from build123d import *

# Parameters (mm, degrees)
F0_R     = 1.5
F1_DEPTH = 5
F2_W     = 5
F2_H     = 5
F2_H_2   = 4.5
F2_R     = 3.5
F3_DEPTH = 3
F4_R     = 1.5
F4_R_2   = 1.4524317573
F5_DEPTH = 25
F6_R     = 3
F7_DEPTH = 7
F8_SIZE  = 1.99999
F9_DEPTH = 25


# Not quite as in the source:
# - a fillet or chamfer is up to 0.001 mm smaller than in the source, because OpenCascade refuses the exact size


with BuildPart() as f1:
    # F0 (on Top) → F1 (new body)
    with BuildSketch(Plane.XY):
        with BuildLine():
            Line((100.4699678509, 5.9815658668), (2.0132142916, 17.3838133968))
            ThreePointArc((2.0132142916, 17.3838133968), (-17.4999985209, -0.0071949455), (2.027507963, -17.3821520952))
            Line((2.027507963, -17.3821520952), (99.6811939192, -5.991524237))
            ThreePointArc((99.6811939192, -5.991524237), (105.987022142, -0.394418396), (100.4699678509, 5.9815658668))
        make_face()
        with BuildLine():
            Line((-11, -8.6602540378), (-2.9686269666, -4.023338655))
            ThreePointArc((-2.9686269666, -4.023338655), (0, -5), (2.9686269666, -4.023338655))
            Line((2.9686269666, -4.023338655), (11, -8.6602540378))
            ThreePointArc((11, -8.6602540378), (0, -14), (-11, -8.6602540378))
        make_face(mode=Mode.SUBTRACT)
        with BuildLine():
            ThreePointArc((-13, -5.1961524227), (-12.124355653, 7), (-2, 13.8564064606))
            Line((-2, 13.8564064606), (-2, 4.582575695))
            ThreePointArc((-2, 4.582575695), (-4.3301270189, 2.5), (-4.9686269666, -0.5592370399))
            Line((-4.9686269666, -0.5592370399), (-13, -5.1961524227))
        make_face(mode=Mode.SUBTRACT)
        Circle(F0_R, mode=Mode.SUBTRACT)
        with BuildLine():
            Line((2, 4.582575695), (2, 13.8564064606))
            ThreePointArc((2, 13.8564064606), (12.124355653, 7), (13, -5.1961524227))
            Line((13, -5.1961524227), (4.9686269666, -0.5592370399))
            ThreePointArc((4.9686269666, -0.5592370399), (4.3301270189, 2.5), (2, 4.582575695))
        make_face(mode=Mode.SUBTRACT)
        with BuildLine():
            Line((30.3816278502, -10.0477205958), (13.8356347618, -11.9776963869))
            ThreePointArc((13.8356347618, -11.9776963869), (18.2999984533, 0.0075238573), (13.8257810711, 11.9890690954))
            Line((13.8257810711, 11.9890690954), (30.3733555452, 10.0726993863))
            ThreePointArc((30.3733555452, 10.0726993863), (31.9999972954, 0.0131564719), (30.3816278502, -10.0477205958))
        make_face(mode=Mode.SUBTRACT)
        with BuildLine():
            Line((67.7617245486, -5.6875905441), (44.2022623135, -8.435639061))
            ThreePointArc((44.2022623135, -8.435639061), (44.9999961967, 0.0185012885), (44.1953109176, 8.4719828198))
            Line((44.1953109176, 8.4719828198), (67.7570248516, 5.743307693))
            ThreePointArc((67.7570248516, 5.743307693), (67.9999942528, 0.0279575027), (67.7617245486, -5.6875905441))
        make_face(mode=Mode.SUBTRACT)
        Polygon((77.8001793809, -5), (77.8001793809, 5), (87.8001793809, 3.8419029556), (87.8001793809, -3.8335690817), align=None, mode=Mode.SUBTRACT)
        with Locations((100, 0)):
            Circle(F0_R, mode=Mode.SUBTRACT)
    extrude(amount=F1_DEPTH)

    # F2 (on face) → F3 (cut)
    with BuildSketch(Plane(origin=(0, 0, 0), x_dir=(1, 0, 0), z_dir=(0, 0, -1))):
        with Locations((38, 6)):
            Rectangle(F2_W, F2_H)
        with Locations((73, 0)):
            Rectangle(F2_W, F2_H_2)
        with Locations((38, -6)):
            Rectangle(F2_W, F2_H)
        with Locations((100, 0)):
            Circle(F2_R)
    extrude(amount=-F3_DEPTH, mode=Mode.SUBTRACT)

    # F4 (on face) → F5 (cut)
    with BuildSketch(Plane.XY.offset(5)):
        with Locations((38, -6)):
            Circle(F4_R)
        with Locations((73, 0)):
            Circle(F4_R)
        with Locations((38, 6)):
            Circle(F4_R_2)
    extrude(amount=-F5_DEPTH, mode=Mode.SUBTRACT)

    # F6 (on face) → F7 (join)
    with BuildSketch(Plane.XY.offset(5)):
        Circle(F6_R)
    extrude(amount=-F7_DEPTH)

    # F8 (size 2 in the source; OpenCascade refuses exactly that, so slightly less here)
    f8_edges = [f1.edges().sort_by_distance(p)[0] for p in [
        (-3, 0, -2),
    ]]
    chamfer(f8_edges, length=F8_SIZE)

    # F9 (cut): a face of the model
    f9_faces = [f1.faces().sort_by_distance(p)[0] for p in [
        (0, 0, -2),
    ]]
    extrude(f9_faces, amount=-F9_DEPTH, mode=Mode.SUBTRACT)


solid = f1.part
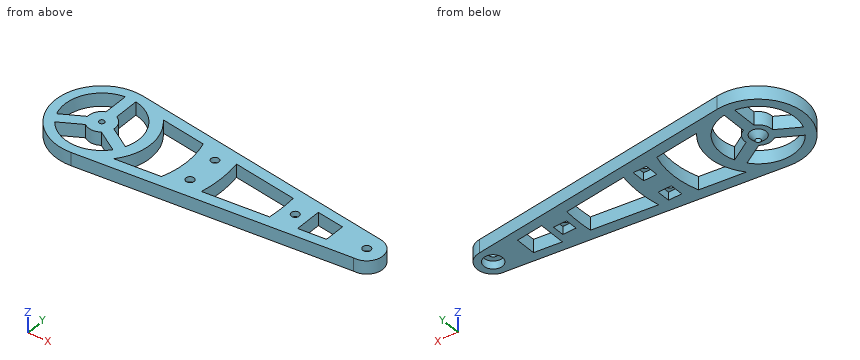
Check sheet for the modelled part. Datum: model origin and axes. Units: mm. Give positions to 0.01 mm unless a question says otherwise; leave off trailing zeros. Write each loop counter-clockwise with the first axis right and the second up, starting at its lowest first coordinate (ties: lowest second). Pieces come first, ordered by that corner, then holes. Notation, with made-up numbers: (65, -1) -> (84, -1) arc R12 ccw to (84, 6) -> close; hole circle Ø7 at (1, 44). An arc over 180 degrees is marked (long way). Use one line per item in the form item = value. Start each with the question number.
1. Go/stop test with flat-tipped pins: P1, Ø0.9, axis at x = 38, z = 1, coming from the -Y side; P2, Ø1.5, axis at x = 73, z = 2, coming from the +Y side; P3, Ø2.5, axis at x = 38.5, z = 1, coming from the +Y side; P4, Ø2.5, axis at x = 38, y = -6, coming from the +Z side. Record where each tip stops, or that it passes through.
2. Thickness scan on line 1 along Y through (x, z) = (-4.5, 3.5); line 2 along X through (y, z) = (3, 4.5); line 3 along X through (y, z) = (-2, 3.75). Record the ranges inside material, lowest first. Write a range as from..to.
3. Section check A-A (x = 24.5). Record the cut outline in (y, z), and give its area (3 significant figures).
4. Section check B-B (z = 1.5). Count the separate pieces of the cut face and the enclosed holes in it, and give its area (3 significant figures).
5. Section check C-C (x = 38). Record the cut outline in (y, z), and give its area (3 significant figures).
6. Section check D-D (x = 73). Record the cut outline in (y, z).
Conclusion:
q1.P1 = -13.24
q1.P2 = 9.25
q1.P3 = 13.3
q1.P4 = through
q2.line_1 = -16.91..-13.26, -4.91..2.18, 13.26..16.91
q2.line_2 = -17.24..-13.67, -4..4, 13.67..18.05, 31.86..44.9, 67.93..77.8, 87.8..105.2
q2.line_3 = -17.39..-13.86, -7.46..7.46, 13.86..18.19, 31.94..44.96, 67.97..77.8, 87.8..105.66
q3.outline = (-14.76, 0) -> (-10.73, 0) -> (-10.73, 5) -> (-14.76, 5) -> close; (10.75, 0) -> (14.78, 0) -> (14.78, 5) -> (10.75, 5) -> close
q3.area = 40.3 mm²
q4.separate_pieces = 1
q4.enclosed_holes = 11
q4.area = 1,630 mm²
q5.outline = (-13.19, 0) -> (-8.5, 0) -> (-8.5, 3) -> (-7.5, 3) -> (-7.5, 5) -> (-13.19, 5) -> close; (-4.5, 3) -> (-3.5, 3) -> (-3.5, 0) -> (3.5, 0) -> (3.5, 3) -> (4.55, 3) -> (4.55, 5) -> (-4.5, 5) -> close; (7.45, 3) -> (8.5, 3) -> (8.5, 0) -> (13.22, 0) -> (13.22, 5) -> (7.45, 5) -> close
q5.area = 90.2 mm²
q6.outline = (-9.1, 0) -> (-2.25, 0) -> (-2.25, 3) -> (-1.5, 3) -> (-1.5, 5) -> (-9.1, 5) -> close; (1.5, 3) -> (2.25, 3) -> (2.25, 0) -> (9.16, 0) -> (9.16, 5) -> (1.5, 5) -> close
